CAD build for the part. Positions are in the model's coordinates, mm. Round coordinates to 2 decimals unless told otherwise and drop trailing zeros. Loops run counter-clockwise (first coordinate to the right, second up) from the corner with the lowest first, then second, coordinate; pieces in that order, holes last. Notation, with made-up numbers: M 50,61.25 L 64,61.25 A25 cw 64,92.25 Z; hole C 66,55.5 d9. An arc over 180 degrees is marked long. Put each result on its own line as item: value. Start each with the question number.
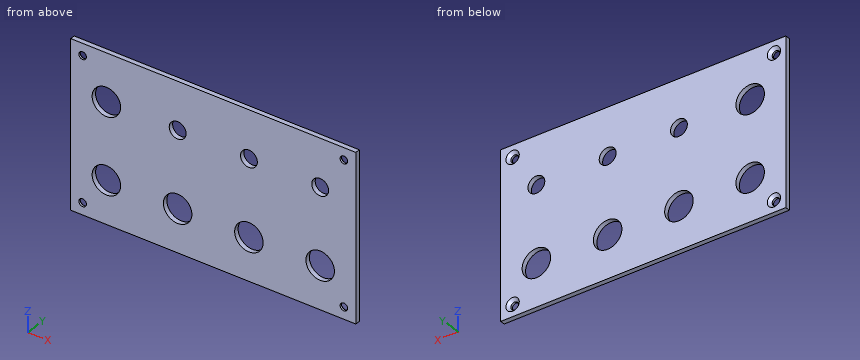
from build123d import *

# Parameters (mm, degrees)
BOTTOM_PLATE_W                       = 120
BOTTOM_PLATE_H                       = 70
BOTTOM_PLATE_EXT_DEPTH               = 2
TOP_ROW_R                            = 6
TOP_ROW_CUT_DEPTH                    = 139.938835464
BOTTOM_ROW_R                         = 3.55
BOTTOM_ROW_R_2                       = 6
BOTTOM_ROW_CUT_DEPTH                 = 139.938835464
PLATE_SCREWS_R                       = 1.6
PLATE_SCREWS_CUT_DEPTH               = 139.938835464
PLATE_SCREW_HEAD_R                   = 2.8
PLATE_SCREW_HEAD_CUT_DEPTH           = 2
PLATE_SCREW_HEAD_CUT_DRAFT           = -45
PLATE_SCREW_HEAD_CUT_PROFILE_2_DEPTH = 2
PLATE_SCREW_HEAD_CUT_PROFILE_2_DRAFT = -45
PLATE_SCREW_HEAD_CUT_PROFILE_3_DEPTH = 2
PLATE_SCREW_HEAD_CUT_PROFILE_3_DRAFT = -45
PLATE_SCREW_HEAD_CUT_PROFILE_4_DEPTH = 2
PLATE_SCREW_HEAD_CUT_PROFILE_4_DRAFT = -45


with BuildPart() as part:
    # Bottom Plate → Bottom Plate EXT (new body)
    with BuildSketch(Plane(origin=(0, 0, 0), x_dir=(1, 0, 0), z_dir=(0, 1, 0))):
        with Locations((-60, 35)):
            Rectangle(BOTTOM_PLATE_W, BOTTOM_PLATE_H)
    extrude(amount=BOTTOM_PLATE_EXT_DEPTH)

    # Top Row → Top Row Cut (cut, through all)
    with BuildSketch(Plane(origin=(0, 2, 0), x_dir=(1, 0, 0), z_dir=(0, 1, 0))):
        with Locations(Location((-105, 52, 0), (0, 0, 270))):
            Circle(TOP_ROW_R)
        with Locations(Location((-75, 52, 0), (0, 0, 270))):
            Circle(TOP_ROW_R)
        with Locations(Location((-45, 52, 0), (0, 0, 270))):
            Circle(TOP_ROW_R)
        with Locations(Location((-15, 52, 0), (0, 0, 270))):
            Circle(TOP_ROW_R)
    extrude(amount=-TOP_ROW_CUT_DEPTH, mode=Mode.SUBTRACT)

    # Bottom Row → Bottom Row Cut (cut, through all)
    with BuildSketch(Plane(origin=(0, 2, 0), x_dir=(1, 0, 0), z_dir=(0, 1, 0))):
        with Locations(Location((-75, 20, 0), (0, 0, 270))):
            Circle(BOTTOM_ROW_R)
        with Locations(Location((-45, 20, 0), (0, 0, 270))):
            Circle(BOTTOM_ROW_R)
        with Locations(Location((-15, 20, 0), (0, 0, 270))):
            Circle(BOTTOM_ROW_R)
        with Locations(Location((-105, 20, 0), (0, 0, 270))):
            Circle(BOTTOM_ROW_R_2)
    extrude(amount=-BOTTOM_ROW_CUT_DEPTH, mode=Mode.SUBTRACT)

    # Plate Screws → Plate Screws Cut (cut, through all)
    with BuildSketch(Plane(origin=(0, 2, 0), x_dir=(1, 0, 0), z_dir=(0, 1, 0))):
        with Locations(Location((-115, 65, 0), (0, 0, 270))):
            Circle(PLATE_SCREWS_R)
        with Locations(Location((-5, 65, 0), (0, 0, 270))):
            Circle(PLATE_SCREWS_R)
        with Locations(Location((-5, 5, 0), (0, 0, 270))):
            Circle(PLATE_SCREWS_R)
        with Locations(Location((-115, 5, 0), (0, 0, 270))):
            Circle(PLATE_SCREWS_R)
    extrude(amount=-PLATE_SCREWS_CUT_DEPTH, mode=Mode.SUBTRACT)


with BuildPart() as plate_screw_head_cut_tool:
    # Plate Screw Head → Plate Screw Head Cut (with draft: the straight prism first)
    with BuildSketch(Plane(origin=(0, 2, 0), x_dir=(1, 0, 0), z_dir=(0, 1, 0))):
        with Locations((-115, 65)):
            Circle(PLATE_SCREW_HEAD_R)
    extrude(amount=-PLATE_SCREW_HEAD_CUT_DEPTH)
    # Plate Screw Head Cut: the draft: its side faces are tilted about the plane it starts from
    plate_screw_head_cut_sides = [plate_screw_head_cut_tool.faces().sort_by_distance(p)[0] for p in [
        (-117.8, 1, -65),
    ]]
    draft(plate_screw_head_cut_sides, Plane(origin=(0, 2, 0), x_dir=(1, 0, 0), z_dir=(0, 1, 0)), PLATE_SCREW_HEAD_CUT_DRAFT)


with BuildPart() as part_1:
    add(part.part)

    # Plate Screw Head Cut: cut by plate_screw_head_cut_tool
    add(plate_screw_head_cut_tool.part, mode=Mode.SUBTRACT)


with BuildPart() as plate_screw_head_cut_profile_2_tool:
    # Plate Screw Head → Plate Screw Head Cut profile 2 (with draft: the straight prism first)
    with BuildSketch(Plane(origin=(0, 2, 0), x_dir=(1, 0, 0), z_dir=(0, 1, 0))):
        with Locations((-5, 65)):
            Circle(PLATE_SCREW_HEAD_R)
    extrude(amount=-PLATE_SCREW_HEAD_CUT_PROFILE_2_DEPTH)
    # Plate Screw Head Cut profile 2: the draft: its side faces are tilted about the plane it starts from
    plate_screw_head_cut_profile_2_sides = [plate_screw_head_cut_profile_2_tool.faces().sort_by_distance(p)[0] for p in [
        (-7.8, 1, -65),
    ]]
    draft(plate_screw_head_cut_profile_2_sides, Plane(origin=(0, 2, 0), x_dir=(1, 0, 0), z_dir=(0, 1, 0)), PLATE_SCREW_HEAD_CUT_PROFILE_2_DRAFT)


with BuildPart() as part_2:
    add(part_1.part)

    # Plate Screw Head Cut profile 2: cut by plate_screw_head_cut_profile_2_tool
    add(plate_screw_head_cut_profile_2_tool.part, mode=Mode.SUBTRACT)


with BuildPart() as plate_screw_head_cut_profile_3_tool:
    # Plate Screw Head → Plate Screw Head Cut profile 3 (with draft: the straight prism first)
    with BuildSketch(Plane(origin=(0, 2, 0), x_dir=(1, 0, 0), z_dir=(0, 1, 0))):
        with Locations((-5, 5)):
            Circle(PLATE_SCREW_HEAD_R)
    extrude(amount=-PLATE_SCREW_HEAD_CUT_PROFILE_3_DEPTH)
    # Plate Screw Head Cut profile 3: the draft: its side faces are tilted about the plane it starts from
    plate_screw_head_cut_profile_3_sides = [plate_screw_head_cut_profile_3_tool.faces().sort_by_distance(p)[0] for p in [
        (-7.8, 1, -5),
    ]]
    draft(plate_screw_head_cut_profile_3_sides, Plane(origin=(0, 2, 0), x_dir=(1, 0, 0), z_dir=(0, 1, 0)), PLATE_SCREW_HEAD_CUT_PROFILE_3_DRAFT)


with BuildPart() as part_3:
    add(part_2.part)

    # Plate Screw Head Cut profile 3: cut by plate_screw_head_cut_profile_3_tool
    add(plate_screw_head_cut_profile_3_tool.part, mode=Mode.SUBTRACT)


with BuildPart() as plate_screw_head_cut_profile_4_tool:
    # Plate Screw Head → Plate Screw Head Cut profile 4 (with draft: the straight prism first)
    with BuildSketch(Plane(origin=(0, 2, 0), x_dir=(1, 0, 0), z_dir=(0, 1, 0))):
        with Locations((-115, 5)):
            Circle(PLATE_SCREW_HEAD_R)
    extrude(amount=-PLATE_SCREW_HEAD_CUT_PROFILE_4_DEPTH)
    # Plate Screw Head Cut profile 4: the draft: its side faces are tilted about the plane it starts from
    plate_screw_head_cut_profile_4_sides = [plate_screw_head_cut_profile_4_tool.faces().sort_by_distance(p)[0] for p in [
        (-117.8, 1, -5),
    ]]
    draft(plate_screw_head_cut_profile_4_sides, Plane(origin=(0, 2, 0), x_dir=(1, 0, 0), z_dir=(0, 1, 0)), PLATE_SCREW_HEAD_CUT_PROFILE_4_DRAFT)


with BuildPart() as part_4:
    add(part_3.part)

    # Plate Screw Head Cut profile 4: cut by plate_screw_head_cut_profile_4_tool
    add(plate_screw_head_cut_profile_4_tool.part, mode=Mode.SUBTRACT)


solid = part_4.part
(1) Cut at B-B on y = 1.7. Count the separate pieces of the cut face and the enclosed holes in it, and give its area (3 significant figures).
(2) Drill centre lines: line 1 along X through (y, z) = (0.3, -5); line 2 along Z through (x, y) = (-5, 0.45); line 3 along X through (y, z) = (1.7, -52.5). Where is each one in solid material? Low to high.
(3) Cut at D-D on z = -5. List the corners of the cut face in (x, y).
(4) Cut at A-A on z = -52. List the corners of the cut face in (x, y).
(5) Cut at C-C on x = -75. List the corners of the cut face in (y, z).
Taken from the geometry:
1. separate pieces: 1
1. enclosed holes: 12
1. area: 7,640 mm2
2. line 1: -120 to -116.6, -113.4 to -6.6, -3.4 to 0
2. line 2: -70 to -66.6, -63.4 to -6.6, -3.4 to 0
2. line 3: -120 to -110.98, -99.02 to -80.98, -69.02 to -50.98, -39.02 to -20.98, -9.02 to 0
3. outline: M -120,0 L -116.6,0 L -116.6,0.8 L -117.8,2 L -120,2 Z; M -113.4,0 L -6.6,0 L -6.6,0.8 L -7.8,2 L -112.2,2 L -113.4,0.8 Z; M -3.4,0 L 0,0 L 0,2 L -2.2,2 L -3.4,0.8 Z
4. outline: M -120,0 L -111,0 L -111,2 L -120,2 Z; M -99,0 L -81,0 L -81,2 L -99,2 Z; M -69,0 L -51,0 L -51,2 L -69,2 Z; M -39,0 L -21,0 L -21,2 L -39,2 Z; M -9,0 L 0,0 L 0,2 L -9,2 Z
5. outline: M 0,-70 L 2,-70 L 2,-58 L 0,-58 Z; M 0,-46 L 2,-46 L 2,-23.55 L 0,-23.55 Z; M 0,-16.45 L 2,-16.45 L 2,0 L 0,0 Z
